from build123d import *

# Parameters (mm, degrees)
F0_W     = 421.2336
F0_H     = 119.9388
F0_R     = 34.5694
F0_R_2   = 29.9974
F1_DEPTH = 12.7


with BuildPart() as f1:
    # F0 (on Front) → F1 (new body)
    with BuildSketch(Plane.XZ):
        with Locations((-4.53439, 5.240247)):
            Rectangle(F0_W, F0_H)
        with Locations((-155.294428, 5.024211)):
            Circle(F0_R, mode=Mode.SUBTRACT)
        with Locations((150.596465, 4.890526)):
            Circle(F0_R_2, mode=Mode.SUBTRACT)
    extrude(amount=-F1_DEPTH)


solid = f1.part
Geometry: final body of the model. Coordinates: model frame, mm. Round coordinates to 2 decimals unless told otherwise and drop trailing zeros. Loops run counter-clockwise (first coordinate to the right, second up) from the corner with the lowest first, then second, coordinate; pieces in that order, holes last.
Q1. Pull-direction query (Z, two-part tool) for faces 1 (the cylindrical face through (120.63, 6.26, 6.21)), 2 (the flat face through (-7, 12.7, 6)), 3 (the flat face through (-7, 6, -54.729)); classes: released by +Z, released by -Z, zero draft, split by the parting line, or undercut.
Q2. Section A-A on x = -132. Return loops of the section in (y, z), plus the area to 3 significant figures.
Q3. Section C-C on x = 134.5. Return loops of the section in (y, z).
Q4. Material intervals for L1, parallel to X at y = 8.75, z = 4; L2, parallel to X at y = 9.5, z = 27; L3, parallel to Z at x = 165.5, y = 3.5, sorted ascending.
Q5. Section D-D on y = 8.25. Return loops of the section in (x, z), plus the area to 3 significant figures.
Q6. Section B-B on z = -12.5. Return loops of the section in (x, y), plus the area to 3 significant figures.
Evaluation:
1. face 1: undercut
1. face 2: zero draft
1. face 3: released by -Z
2. outline: (0, -54.73) - (12.7, -54.73) - (12.7, -20.52) - (0, -20.52) - close; (0, 30.57) - (12.7, 30.57) - (12.7, 65.21) - (0, 65.21) - close
2. area: 874 mm2
3. outline: (0, -54.73) - (12.7, -54.73) - (12.7, -20.42) - (0, -20.42) - close; (0, 30.2) - (12.7, 30.2) - (12.7, 65.21) - (0, 65.21) - close
4. L1: x = -215.15 to -189.85, -120.74 to 120.61, 180.58 to 206.08
4. L2: x = -215.15 to -181.98, -128.61 to 130.32, 170.87 to 206.08
4. L3: z = -54.73 to -21.14, 30.92 to 65.21
5. outline: (-215.15, -54.73) - (206.08, -54.73) - (206.08, 65.21) - (-215.15, 65.21) - close; hole circle Ø69.14 at (-155.29, 5.02); hole circle Ø59.99 at (150.6, 4.89)
5. area: 43,900 mm2
6. outline: (-215.15, 0) - (-185.09, 0) - (-185.09, 12.7) - (-215.15, 12.7) - close; (-125.5, 0) - (126.15, 0) - (126.15, 12.7) - (-125.5, 12.7) - close; (175.04, 0) - (206.08, 0) - (206.08, 12.7) - (175.04, 12.7) - close
6. area: 3,970 mm2
